Autodesk Inventor part; units mm, degrees
ref_plane "YZ Plane" through (0, 0, 0) normal (1, 0, 0) x (0, 1, 0)
ref_plane "XZ Plane" through (0, 0, 0) normal (0, 1, 0) x (-1, 0, 0)
ref_plane "XY Plane" through (0, 0, 0) normal (0, 0, 1) x (1, 0, 0)
sketch "Sketch1" plane through (0, 0, 0) normal (0, 1, 0) x (-1, 0, 0)
  line L0 (0, 0) -> (-63.5, 0)
  line L1 (-63.5, 0) -> (-63.5, -63.5)
  line L2 (-63.5, -63.5) -> (0, -63.5)
  line L3 (0, -63.5) -> (0, 0)
  line L4 (-63.5, -57.15) -> (-63.5, -63.5)
  line L5 (-63.5, -6.35) -> (-63.5, 0)
  line L6 (-63.5, -31.75) -> (-63.5, -41.656)
  line L7 (-63.5, -31.75) -> (-63.5, -21.844)
  line L8 (-63.5, -21.844) -> (-81.4578, -21.844)
  line L9 (-81.4578, -21.844) -> (-81.4578, -15.494)
  line L10 (-81.4578, -15.494) -> (-63.5, -15.494)
  line L11 (-63.5, -15.494) -> (-63.5, -21.844)
  line L12 (-63.5, -41.656) -> (-81.4578, -41.656)
  line L13 (-81.4578, -41.656) -> (-81.4578, -48.006)
  line L14 (-81.4578, -48.006) -> (-63.5, -48.006)
  line L15 (-63.5, -48.006) -> (-63.5, -41.656)
  line L16 (0, 0) -> (-1.7961, -1.7961)
  line L17 (0, 0) -> (2.54, 0) construction
  line L18 (-63.5, -63.5) -> (-61.7039, -61.7039)
  line L19 (-1.7961, -1.7961) -> (-61.7039, -1.7961)
  line L20 (-61.7039, -1.7961) -> (-61.7039, -61.7039)
  line L21 (-61.7039, -61.7039) -> (-1.7961, -61.7039)
  line L22 (-1.7961, -61.7039) -> (-1.7961, -1.7961)
  point P0 (-63.5, -15.494)
  dimension "PlatformL" = 63.5
  dimension "PlatformW" = 63.5
  dimension "SideThickness" = 9.906
  dimension "d12" = 9.906
  dimension "EarWidth" = 17.9578
  dimension "EarThickness" = 6.35
  dimension "d15" = 17.9578
  dimension "d16" = 6.35
  dimension "d26" = 2.54
  dimension "d27" = 135
  dimension "d28" = 2.54
extrude "Extrusion1" add sketch "Sketch1" along normal blind 6.35 contours L22 L21 L20 L19
extrude "Extrusion2" add sketch "Sketch1" along normal blind 57.15 contours L1 L8 L9 L10 | L14 L13 L12 L1
sketch "Sketch3" plane through (63.5, 0, -15.494) normal (0, 0, 1) x (1, 0, 0)
  line L0 (0, 0) -> (17.9578, 0)
  line L1 (8.9789, 0) -> (8.9789, 50.8)
  line L2 (8.9789, 0) -> (59.7789, 0) construction
  point P0 (-63.5, 0)
  dimension "HeightToHole" = 50.8
  dimension "d18" = 90
hole "Hole1" at (72.4789, 50.8, -15.494) direction (0, 0, -1) diameter 6.7564 end through all
extrude "Extrusion3" add sketch "Sketch1" along normal blind 7.62 contours L16 L19 L20 L18 L1 L0 | L3 L2 L18 L21 L22 L16
equation "\"d12\" = SideThickness"
equation "\"d15\" = EarWidth"
equation "\"d16\" = EarThickness"
properties part number "wastebottleholder"
Check sheet for the modelled part. Datum: model origin and axes. Units: mm. A direction names the side the tool comes from. Give positions to 0.01 mm unless a question says otherwise; leave off trailing zeros. Loops run counter-clockwise (first coordinate to the right, second up) from the corner with the lowest first, then second, coordinate; pieces in that order, holes last. Notation, with made-up numbers: M 86,74.25 L 123,74.25 A12 ccw 123,86.25 Z; hole C 71,70 d6. An arc over 180 degrees is marked long. Answer as CSV lines item,"result".
Item 1: Sectioned sample at C-C, the plane x = 17.5. Enter the section's corners in (y, z), then the cut area to 3 significant figures.
Reply:
outline,"M 0,-63.5 L 7.62,-63.5 L 7.62,-61.7 L 6.35,-61.7 L 6.35,-1.8 L 7.62,-1.8 L 7.62,0 L 0,0 Z"
area,"408 mm^2"
Item 2: Depth check by flat-ended pin: pin 1 Ø8.5 at (y, z) = (5.5, -34) entering from +X; pin 2 Ø5.5 at (x, y) = (68.5, 31) entering from +Z; pin 3 Ø10 at (x, z) = (28.5, -56) entering from +Y. Enter the tip coordinate at first touch or a pass-through.
Reply:
pin 1,"x = 63.5"
pin 2,"z = -15.49"
pin 3,"y = 6.35"
Item 3: Scan lines: L1, parallel to X at y = 50.8, z = -18.5; L2, parallel to Z at x = 76.5, y = 9.5; L3, parallel to Z at x = 8.5, y = 6.5. Record each from-to range of solid material in increasing order.
Reply:
L1,"63.5 to 69.1, 75.86 to 81.46"
L2,"-48.01 to -41.66, -21.84 to -15.49"
L3,"-63.5 to -61.7, -1.8 to 0"
Item 4: Sectioned sample at D-D, the plane z = -46.5. Enter the section's corners in (x, y).
Reply:
outline,"M 0,0 L 81.46,0 L 81.46,57.15 L 63.5,57.15 L 63.5,7.62 L 61.7,7.62 L 61.7,6.35 L 1.8,6.35 L 1.8,7.62 L 0,7.62 Z; hole C 72.48,50.8 d6.76"
Item 5: Set-up check for faces 5 (the face through (63.5, 32, -19)), 6 (the face through (63.5, 4, -8)), 7 (the face through (32, 6.35, -31)), 8 (the face through (73, 57.15, -19)): record each of +Z, -Z, +X, -X, +Y, -Y from which the full face is reachable in a straight line by a thin tool's end or side.
Reply:
face 5,"+Z, -Z, -X, +Y"
face 6,"+Z, +X, +Y, -Y"
face 7,"+Y"
face 8,"+Z, -Z, +X, -X, +Y"
Item 6: Draft check along X on faces 1 (the face through (63.5, 4, -32)), 2 (the face through (71.46, 47.58, -18.71)), 3 (the face through (0, 4, -32)), 4 (the face through (72, 28, -41.656)). Enter one of: pulls with the +X half, pulls with the -X half, needs draft (parallel to the pull), parting line crosses it, or undercut.
Reply:
face 1,"pulls with the +X half"
face 2,"undercut"
face 3,"pulls with the -X half"
face 4,"needs draft"
Item 7: Sectioned sample at A-A, the plane y = 21. Enter the section's corners in (x, z).
Reply:
outline,"M 63.5,-48.01 L 81.46,-48.01 L 81.46,-41.66 L 63.5,-41.66 Z; M 63.5,-21.84 L 81.46,-21.84 L 81.46,-15.49 L 63.5,-15.49 Z"
Item 8: Sectioned sample at B-B, the plane y = 50.8. Enter the section's corners in (x, z).
Reply:
outline,"M 63.5,-48.01 L 69.1,-48.01 L 69.1,-41.66 L 63.5,-41.66 Z; M 63.5,-21.84 L 69.1,-21.84 L 69.1,-15.49 L 63.5,-15.49 Z; M 75.86,-48.01 L 81.46,-48.01 L 81.46,-41.66 L 75.86,-41.66 Z; M 75.86,-21.84 L 81.46,-21.84 L 81.46,-15.49 L 75.86,-15.49 Z"
